from build123d import *

# Parameters (mm, degrees)
F2_ANGLE = 90
F3_DEPTH = 65


with BuildPart() as f2:
    # F1 (on Top) → F2 (revolve)
    with BuildSketch(Plane.XY):
        Polygon((90, -10), (90, 0), (67.5, 0), align=None)
    revolve(axis=Axis((65, 13.2645983249, 0), (0, -1, 0)), revolution_arc=F2_ANGLE)

    # F3 (add): a face of the model
    f3_faces = [f2.faces().sort_by_distance(p)[0] for p in [
        (65, -3.3333333333, 17.5),
    ]]
    extrude(f3_faces, amount=F3_DEPTH)

    # F4: F2 across plane


with BuildPart() as f2_1:
    add(f2.part)
    add(f2.part.mirror(Plane.YZ))


solid = f2_1.part
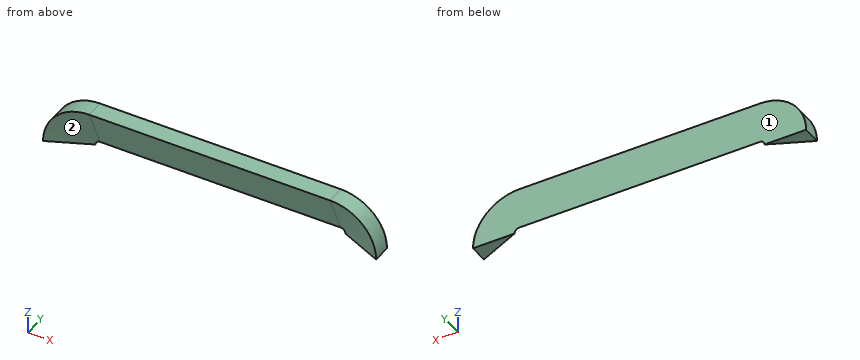
Geometry: final body of the model. Coordinates: model frame, mm. Face numbers are marked on the shaded views. Round coordinates to 2 decimals unless told otherwise and drop trailing zeros. Loops run counter-clockwise (first coordinate to the right, second up) from the corner with the lowest first, then second, coordinate; pieces in that order, holes last. Notation, with made-up numbers: (20, 77) -> (67, 77) arc R12 cw to (67, 88) -> close; hole circle Ø8 at (-32.75, 63). An arc over 180 degrees is marked (long way). One line per question, with ' | ' between items. Start each with the question number.
1. Line query: line 1 along X through (y, z) = (-5.25, 2.25); line 2 along X through (y, z) = (-1, 2); line 3 along X through (y, z) = (-1.25, 14). Output: solid intervals per line, ascending. Write a range as [from, to].
2. Section A-A on y = -3. Output: boundary loops of the cut face in (x, z), and give its area (3 significant figures).
3. Section B-B on x = 21.5. Output: boundary loops of the cut face in (y, z).
4. Mould query, pull axis X, two halves, no side actions, for the marked faces 1 and 2. Classes: pulls with the +X half, pulls with the -X half, needs draft (parallel to the pull), parting line crosses it, or undercut.
5. Contact query for flat-ended pins moving along their axis: pin 1 (4 mm diameter, centred on x = -9, z = 17, fed in from +Y); pin 2 (4 mm diameter, centred on y = -7, z = 21.5, fed in from -X); pin 3 (1.5 mm diameter, centred on y = -5.5, z = 7, fed in from +X). Output: stop coordinate, or through.
Returned:
1) line 1: x = [-89.9, -79.13], [79.13, 89.9] | line 2: x = [-89.92, -69.31], [69.31, 89.92] | line 3: x = [-85.71, 85.71]
2) outline: (-90, 0) -> (-74.25, 0) arc R9.25 cw to (-65, 9.25) -> (65, 9.25) arc R9.25 cw to (74.25, 0) -> (90, 0) arc R25 ccw to (65, 25) -> (-65, 25) arc R25 ccw to start | area: 2,890 mm2
3) outline: (-10, 25) -> (0, 2.5) -> (0, 25) -> close
4) face 1: needs draft | face 2: undercut
5) pin 1: stops at y = 0 | pin 2: stops at x = -80.64 | pin 3: stops at x = 89.21
